from build123d import *

# Parameters (mm, degrees)
F0_R     = 152.4
F1_DEPTH = 50.8
F2_R     = 12.7
F3_R     = 4.733827
F4_DEPTH = 25.4


with BuildPart() as f1:
    # F0 (on Top) → F1 (new body)
    with BuildSketch(Plane.XY):
        Circle(F0_R)
    extrude(amount=F1_DEPTH)

    # F2
    f2_edges = [f1.edges().sort_by_distance(p)[0] for p in [
        (-152.4, 0, 50.8),
        (-152.4, 0, 0),
    ]]
    fillet(f2_edges, radius=F2_R)

    # F3 (on face) → F4 (cut)
    with BuildSketch(Plane.XY.offset(50.8)):
        with Locations((-94.924906, -9.525)):
            Circle(F3_R)
        with Locations((-94.924906, 9.525)):
            Circle(F3_R)
        with Locations((-76.2, 0)):
            Circle(F3_R)
        with Locations((-9.53826, -94.923999)):
            Circle(F3_R)
        with Locations((0, -76.2)):
            Circle(F3_R)
        with Locations((9.53826, -94.923999)):
            Circle(F3_R)
        with Locations((76.2, 0)):
            Circle(F3_R)
        with Locations((94.924906, 9.525)):
            Circle(F3_R)
        with Locations((94.924906, -9.525)):
            Circle(F3_R)
        with Locations((0, 76.2)):
            Circle(F3_R)
        with Locations((9.525, 94.924906)):
            Circle(F3_R)
        with Locations((-9.525, 94.924906)):
            Circle(F3_R)
    extrude(amount=-F4_DEPTH, mode=Mode.SUBTRACT)


solid = f1.part
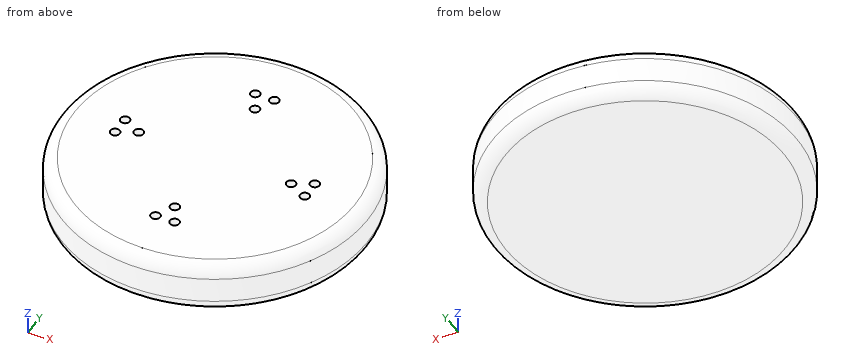
Part model, mm, in its own coordinate system. Coordinates: 2 decimals unless noted, no trailing zeros. Loops run counter-clockwise (first coordinate to the right, second up) from the corner with the lowest first, then second, coordinate; pieces in that order, holes last. Notation, with made-up numbers: (63.5, -10.5) - (93.5, -10.5) arc R23 ccw to (93.5, 23.5) - close; hole circle Ø6 at (26.5, 75). An arc over 180 degrees is marked (long way). Write each question's results on one line, items separated by ' | '. Start each with the question number.
Q1. Slice it at A-A on x = 0. Give the cut face in (y, z), and give its area (3 significant figures).
Q2. Slice it at D-D on z = 20.5. Give the cut face in (x, y).
Q3. Slice it at C-C on z = 42. Give the number of separate pieces and of enclosed holes in the cut face, and give its area (3 significant figures).
Q4. Drop flat-ended pins along their axis: pin 1 Ø3 at (x, y) = (-97, -11) entering from +Z; pin 2 Ø6 at (y, z) = (71, 45.5) entering from -X; pin 3 Ø3 at (x, z) = (24, 33.5) entering from -Y. Give the stop position or say it passes through.
Q5. Probe line 1 along Y through (x, z) = (0, 34); line 2 along Y through (x, z) = (95.5, 47); line 3 along Y through (x, z) = (-76.2, 36). List the from-to ranges inside material, lowest first.
Answer:
1) outline: (-152.4, 12.7) arc R12.7 ccw to (-139.7, 0) - (139.7, 0) arc R12.7 ccw to (152.4, 12.7) - (152.4, 38.1) arc R12.7 ccw to (139.7, 50.8) - (80.93, 50.8) - (80.93, 25.4) - (71.47, 25.4) - (71.47, 50.8) - (-71.47, 50.8) - (-71.47, 25.4) - (-80.93, 25.4) - (-80.93, 50.8) - (-139.7, 50.8) arc R12.7 ccw to (-152.4, 38.1) - close | area: 14,900 mm2
2) outline: circle Ø304.8 at (0, 0)
3) separate pieces: 1 | enclosed holes: 12 | area: 71,500 mm2
4) pin 1: stops at z = 25.4 | pin 2: stops at x = -134.66 | pin 3: stops at y = -150.73
5) line 1: y = -152.4 to -80.93, -71.47 to 71.47, 80.93 to 152.4 | line 2: y = -114.06 to -14.22, -4.83 to 4.83, 14.22 to 114.06 | line 3: y = -131.98 to -4.73, 4.73 to 131.98
